Autodesk Inventor part; units mm, degrees
ref_plane "YZ Plane" through (0, 0, 0) normal (1, 0, 0) x (0, 1, 0)
ref_plane "XZ Plane" through (0, 0, 0) normal (0, 1, 0) x (-1, 0, 0)
ref_plane "XY Plane" through (0, 0, 0) normal (0, 0, 1) x (1, 0, 0)
sketch "Szkic1" plane through (0, 0, 0) normal (0, 1, 0) x (-1, 0, 0)
  line L0 (0, 0) -> (7.5, 0)
  line L1 (0, 0) -> (7.5, 0) construction
  circle A0 centre (7.5, 0) radius 2.2
  line L2 (0, 0) -> (0, -2)
  circle A1 centre (-7.5, 0) radius 2.2
  line L3 (-38.5, 38.5) -> (38.5, 38.5)
  line L4 (38.5, 38.5) -> (38.5, -38.5)
  line L5 (38.5, -38.5) -> (-38.5, -38.5)
  line L6 (-38.5, -38.5) -> (-38.5, 38.5)
  line L7 (-38.5, 38.5) -> (38.5, -38.5) construction
  line L8 (38.5, 38.5) -> (-38.5, -38.5) construction
  circle A2 centre (7.5, 0) radius 3.5
  circle A3 centre (-7.5, 0) radius 3.5
  dimension "d0" = 7.5
  dimension "d1" = 0
  dimension "d2" = 4.4
  dimension "d3" = 2
  dimension "d4" = 77
  dimension "d5" = 77
  dimension "d8" = 7
extrude "Wyciągnięcie proste1" add sketch "Szkic1" along normal blind 6 contours A2 | L3 L4 L5 L6 | A3
extrude "Wyciągnięcie proste2" cut sketch "Szkic1" along normal blind 3 contours A2 | A3
chamfer "Faza1" distance 2 angle 45 4 edges at (-38.5, 0, 0) (0, 0, -38.5) (38.5, 0, 0) (0, 0, 38.5)
sketch "Szkic2" plane through (0, 6, 0) normal (0, 1, 0) x (1, 0, 0)
  line L0 (12.5, -5) -> (-12.5, -5)
  line L1 (-12.5, -5) -> (-12.5, 5)
  line L2 (-12.5, 5) -> (12.5, 5)
  line L3 (12.5, 5) -> (12.5, -5)
  line L4 (12.5, -5) -> (-12.5, 5) construction
  line L5 (-12.5, -5) -> (12.5, 5) construction
  circle A0 centre (-7.5, 0) radius 2.2
  circle A1 centre (-7.5, 0) radius 2.2
  circle A2 centre (7.5, 0) radius 2.2
  circle A3 centre (7.5, 0) radius 2.2
  point P0 (0, 0)
  dimension "d14" = 25
  dimension "d15" = 10
extrude "Wyciągnięcie proste3" add sketch "Szkic2" along normal blind 4
chamfer "Faza2" distance 4 angle 45 4 edges at (0, 6, 5) (12.5, 6, 0) (0, 6, -5) (-12.5, 6, 0)
properties part number "taca"
Verification items for the finished model (mm, model axes). A direction names the side the tool comes from. Give positions to 0.01 mm unless a question says otherwise; leave off trailing zeros. Write each loop counter-clockwise with the first axis right and the second up, starting at its lowest first coordinate (ties: lowest second). Pieces come first, ordered by that corner, then holes. Notation, with made-up numbers: (67.5, 65.5) - (106.5, 65.5) arc R10 cw to (106.5, 74.5) - close; hole circle Ø8 at (87.5, -31.5). An arc over 180 degrees is marked (long way). Answer as CSV lines item,"result". Start each with the question number.
1. Draft check along Z on faces 1 (the face through (38.5, 4, -1)), 2 (the face through (-4, 1, 0)), 3 (the face through (0, 8, 7)). Enter one of: pulls with the +Z half, pulls with the -Z half, needs draft (parallel to the pull), parting line crosses it, or undercut.
2. Sectioned sample at A-A (z = 0). Count the separate pieces of the cut face and the enclosed holes in it, then the cut area to 3 significant figures.
3. Set-up check for faces 4 (the face through (9, 3, -2)), 5 (the face through (-0.5, 1, -37.5)): record each of +Z, -Z, +X, -X, +Y, -Y from which the full face is reachable in a straight line by a thin tool's end or side.
4. Thickness scan on line 1 (X direction, y = 4.5, z = 0); line 2 (X direction, y = 7.25, z = 0); line 3 (Y direction, x = -15.5, z = 28). Record the ranges inside material, lowest first.
5. Sectioned sample at D-D (z = -26). Record the boundary of the cut face in (x, y).
6. Depth check by flat-ended pin: pin 1 (11 mm diameter, centred on x = -7.5, z = 0, fed in from +Y); pin 2 (2 mm diameter, centred on x = -4, z = 26.5, fed in from +Y); pin 3 (1.5 mm diameter, centred on x = 8.5, y = 7, fed in from +Z). Enter the tip coordinate at first touch or a pass-through.
7. Sectioned sample at C-C (x = -28). Record the boundary of the cut face in (y, z), then the cut area to 3 significant figures.
Derived:
1,face 1,"needs draft"
1,face 2,"undercut"
1,face 3,"pulls with the +Z half"
2,separate pieces,"3"
2,enclosed holes,"0"
2,area,"470 mm²"
3,face 4,"-Y"
3,face 5,"-Z, +X, -X, -Y"
4,line 1,"-38.5 to -9.7, -5.3 to 5.3, 9.7 to 38.5"
4,line 2,"-15.25 to -9.7, -5.3 to 5.3, 9.7 to 15.25"
4,line 3,"0 to 6"
5,outline,"(-38.5, 2) - (-36.5, 0) - (36.5, 0) - (38.5, 2) - (38.5, 6) - (-38.5, 6) - close"
6,pin 1,"y = 10"
6,pin 2,"y = 6"
6,pin 3,"z = 8.75"
7,outline,"(0, -36.5) - (2, -38.5) - (6, -38.5) - (6, 38.5) - (2, 38.5) - (0, 36.5) - close"
7,area,"458 mm²"
